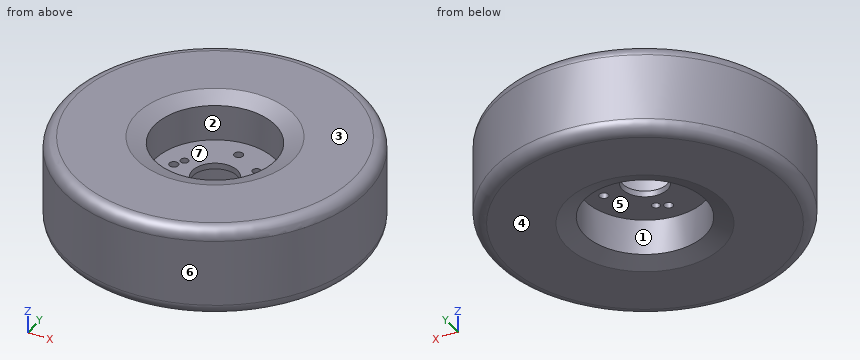
from build123d import *
from OCP.BRepFilletAPI import BRepFilletAPI_MakeChamfer

# Parameters (mm, degrees)
SKETCH1_R                            = 127
SKETCH1_R_2                          = 50.8
BOSS_EXTRUDE1_DEPTH                  = 38.1
CHAMFER1_SIZE                        = 15
CHAMFER1_SIZE2                       = 5.459553514
FILLET1_R                            = 10
SKETCH2_R                            = 50.8
SKETCH2_R_2                          = 19.05
BOSS_EXTRUDE2_DEPTH                  = 2.5
F_19_64_0_29688_DIAMETER_HOLE1_D     = 7.540752
F_19_64_0_29688_DIAMETER_HOLE1_DEPTH = 18.75
F_19_64_0_29688_DIAMETER_HOLE1_TIP   = 2.265470457
F_1_4_CLEARANCE_HOLE1_D              = 6.7564
F_1_4_CLEARANCE_HOLE1_DEPTH          = 18.75
F_1_4_CLEARANCE_HOLE1_TIP            = 2.029827343


with BuildPart() as part:
    # Sketch1 → Boss-Extrude1 (new, symmetric)
    with BuildSketch(Plane.XY):
        with Locations(Location((0, 0, 0), (0, 0, 180))):
            Circle(SKETCH1_R)
        with Locations(Location((0, 0, 0), (0, 0, 180))):
            Circle(SKETCH1_R_2, mode=Mode.SUBTRACT)
    extrude(amount=BOSS_EXTRUDE1_DEPTH, both=True)

    # Chamfer1: one chamfer whose edges measure the first distance from different faces: ONE call of the kernel's chamfer builder (chamfer() names one face for all edges)
    chamfer1_edges_1 = [part.edges().sort_by_distance(p)[0] for p in [
        (50.8, 0, -38.1),
    ]]
    chamfer1_side_1 = [part.faces().sort_by_distance(p)[0] for p in [
        (123.407897552, 0, -38.1),
    ]]
    chamfer1_edges_2 = [part.edges().sort_by_distance(p)[0] for p in [
        (50.8, 0, 38.1),
    ]]
    chamfer1_side_2 = [part.faces().sort_by_distance(p)[0] for p in [
        (123.407897552, 0, 38.1),
    ]]
    chamfer1 = BRepFilletAPI_MakeChamfer(part.part.solid().wrapped)
    for e in chamfer1_edges_1:
        chamfer1.Add(CHAMFER1_SIZE, CHAMFER1_SIZE2, e.wrapped, chamfer1_side_1[0].wrapped)  # the first distance lies on this face
    for e in chamfer1_edges_2:
        chamfer1.Add(CHAMFER1_SIZE, CHAMFER1_SIZE2, e.wrapped, chamfer1_side_2[0].wrapped)  # the first distance lies on this face
    add(Compound.cast(chamfer1.Shape()), mode=Mode.REPLACE)

    # Fillet1
    fillet1_edges = [part.edges().sort_by_distance(p)[0] for p in [
        (127, 0, -38.1),
        (127, 0, 38.1),
    ]]
    fillet(fillet1_edges, radius=FILLET1_R)

    # Sketch2 → Boss-Extrude2 (add, symmetric)
    with BuildSketch(Plane.XY):
        with Locations(Location((0, 0, 0), (0, 0, 180))):
            Circle(SKETCH2_R)
        Circle(SKETCH2_R_2, mode=Mode.SUBTRACT)
    extrude(amount=BOSS_EXTRUDE2_DEPTH, both=True)

    # 19/64 (0.29688) Diameter Hole1
    with Locations(Plane.XY.offset(2.5)):
        with Locations((0, 35.052), (35.052, 0), (0, -35.052), (-35.052, 0)):
            Hole(F_19_64_0_29688_DIAMETER_HOLE1_D / 2, depth=F_19_64_0_29688_DIAMETER_HOLE1_DEPTH)
            with Locations((0, 0, -(F_19_64_0_29688_DIAMETER_HOLE1_DEPTH + F_19_64_0_29688_DIAMETER_HOLE1_TIP / 2))):  # 118° drill point
                Cone(0, F_19_64_0_29688_DIAMETER_HOLE1_D / 2, F_19_64_0_29688_DIAMETER_HOLE1_TIP, mode=Mode.SUBTRACT)

    # 1/4 Clearance Hole1
    with Locations(Plane.XY.offset(2.5)):
        with Locations((-30.668144985, 8.217504682), (22.450640303, 22.450640303), (8.217504682, -30.668144985)):
            Hole(F_1_4_CLEARANCE_HOLE1_D / 2, depth=F_1_4_CLEARANCE_HOLE1_DEPTH)
            with Locations((0, 0, -(F_1_4_CLEARANCE_HOLE1_DEPTH + F_1_4_CLEARANCE_HOLE1_TIP / 2))):  # 118° drill point
                Cone(0, F_1_4_CLEARANCE_HOLE1_D / 2, F_1_4_CLEARANCE_HOLE1_TIP, mode=Mode.SUBTRACT)


solid = part.part
Can you work these out from the model? Positions are in its coordinate system, mm. Face numbers are marked on the shaded views. A direction names the side the tool comes from. Give positions to 0.01 mm unless a question says otherwise; leave off trailing zeros. Loops run counter-clockwise (first coordinate to the right, second up) from the corner with the lowest first, then second, coordinate; pieces in that order, holes last. Notation, with made-up numbers: (-20.5, 10.25) -> (36.5, 10.25) arc R33 ccw to (36.5, 40.25) -> close; hole circle Ø7 at (4, 75.5). An arc over 180 degrees is marked (long way). Return JSON: item names as keys, results as strings.
Q1. On a 3-axis mill with a long thin cutter (end or side, diameter ignored), from which of +Z, -Z, +X, -X, +Y, -Y can I reach the whole of each face in a straight line? I mean the marked faces 1, 2 and 3. Say none if no direction works.
Checks:
{"face 1": "-Z", "face 2": "+Z", "face 3": "+Z, +X, -X, +Y, -Y"}
Q2. I want a section at C-C, the plane z = 8. List the corners of the cut face in (x, y) for me.
Checks:
{"outline": "circle Ø254 at (0, 0); hole circle Ø101.6 at (0, 0)"}
Q3. I want a section at A-A, the plane y = 0. Count the separate pieces of the cut face and the enclosed holes in it, then the cut area to 3 significant figures.
Checks:
{"separate pieces": "4", "enclosed holes": "0", "area": "11,600 mm2"}
Q4. I need wall thicknesses on probe 1 along Y at (x, z) = (0, -0.9); probe 2 along X at (y, z) = (-13, -26); probe 3 along Y at (x, z) = (9, 20.5). Which ranges of each line are inside material? Lowest first, please.
Checks:
{"probe 1": "y = -127 to -38.82, -31.28 to -19.05, 19.05 to 31.28, 38.82 to 127", "probe 2": "x = -126.33 to -49.11, 49.11 to 126.33", "probe 3": "y = -126.68 to -50, 50 to 126.68"}
Q5. We'd pull the mould along X, two halves only. Please class the marked faces 4, 5, 6 and 7: released by +X, released by -X, zero draft, split by the parting line, or undercut.
Checks:
{"face 4": "zero draft", "face 5": "undercut", "face 6": "split by the parting line", "face 7": "undercut"}
Q6. For pin 1 Ø8 at (x, z) = (-98.5, 27.5) entering from -Y; pin 2 Ø8 at (x, y) = (-30.67, 8.22) entering from -Z; pin 3 Ø12 at (x, y) = (-48.5, -16.5) entering from -Z, each with a flat end and sliding along its axis, tell me the tip position at first contact or that it passes through.
Checks:
{"pin 1": "stops at y = -84.85", "pin 2": "stops at z = -2.5", "pin 3": "stops at z = -34.98"}
